Verification items for the finished model (mm, model axes). A direction names the side the tool comes from. Give positions to 0.01 mm unless a question says otherwise; leave off trailing zeros. Loops run counter-clockwise (first coordinate to the right, second up) from the corner with the lowest first, then second, coordinate; pieces in that order, holes last. Notation, with made-up numbers: M -39.5,-3 L 12.5,-3 A16 ccw 12.5,14 Z; hole C 11,21.5 d9. An arc over 180 degrees is marked long. Use CSV: the item, a comma, the result in double quotes.
from build123d import *

# Parameters (mm, degrees)
CROQUIS1_W              = 42
CROQUIS1_H              = 33.5
SALIENTE_EXTRUIR1_DEPTH = 5.5
SALIENTE_EXTRUIR2_DEPTH = 12
NERVIO4_REACH           = 72.794
CROQUIS4_WALL_W         = 160.558874412
CROQUIS4_WALL_H         = 8
CROQUIS5_R              = 4.5
CORTAR_EXTRUIR1_DEPTH   = 12
CROQUIS6_R              = 11.3
CORTAR_EXTRUIR2_DEPTH   = 9
CORTAR_EXTRUIR3_DEPTH   = 70.507193872
CHAFL_N1_SIZE           = 5


with BuildPart() as part:
    # Croquis1 → Saliente-Extruir1 (new, symmetric)
    with BuildSketch(Plane.XY):
        Rectangle(CROQUIS1_W, CROQUIS1_H)
        Polygon((21, -16.75), (-21, -16.75), (-45, -16.75), (-45, -33.25), (45, -33.25), (45, -16.75), align=None)
    extrude(amount=SALIENTE_EXTRUIR1_DEPTH, both=True)

    # Croquis2 → Saliente-Extruir2 (add)
    with BuildSketch(Plane.XY.offset(5.5)):
        Polygon((-21, -16.75), (-45, -16.75), (-45, -33.25), (45, -33.25), (45, -16.75), (21, -16.75), align=None)
    extrude(amount=SALIENTE_EXTRUIR2_DEPTH)

    # Croquis4 wall → Nervio4 (add, up to next)
    with BuildSketch(Plane(origin=(15, -10.75, 11.5), x_dir=(0, -0.707106781187, 0.707106781187), z_dir=(0, -0.707106781187, -0.707106781187)), mode=Mode.PRIVATE) as nervio4_sk1:
        Rectangle(CROQUIS4_WALL_W, CROQUIS4_WALL_H)
    nervio4_tool1 = extrude(nervio4_sk1.sketch, amount=NERVIO4_REACH, mode=Mode.PRIVATE) - part.part
    nervio4 = nervio4_tool1.solids().sort_by_distance((15, -10.75, 11.5))[0]
    add(nervio4)

    # Simetría1: Nervio4 across plane
    add(nervio4.mirror(Plane(origin=(0, 0, 0), x_dir=(0, 0, 1), z_dir=(1, 0, 0))))

    # Croquis5 → Cortar-Extruir1 (cut)
    with BuildSketch(Plane.XY.offset(5.5)):
        Circle(CROQUIS5_R)
    extrude(amount=-CORTAR_EXTRUIR1_DEPTH, mode=Mode.SUBTRACT)

    # Croquis6 → Cortar-Extruir2 (cut)
    with BuildSketch(Plane.XY.offset(5.5)):
        Circle(CROQUIS6_R)
    extrude(amount=-CORTAR_EXTRUIR2_DEPTH, mode=Mode.SUBTRACT)

    # Croquis7 → Cortar-Extruir3 (cut, through all)
    with BuildSketch(Plane.XZ.offset(33.25)):
        with BuildLine():
            Line((-38.5, 8.5), (-26.5, 8.5))
            ThreePointArc((-26.5, 8.5), (-24, 6), (-26.5, 3.5))
            Line((-26.5, 3.5), (-38.5, 3.5))
            ThreePointArc((-38.5, 3.5), (-41, 6), (-38.5, 8.5))
        make_face()
        with BuildLine():
            Line((38.5, 8.5), (26.5, 8.5))
            ThreePointArc((26.5, 8.5), (24, 6), (26.5, 3.5))
            Line((26.5, 3.5), (38.5, 3.5))
            ThreePointArc((38.5, 3.5), (41, 6), (38.5, 8.5))
        make_face()
    extrude(amount=-CORTAR_EXTRUIR3_DEPTH, mode=Mode.SUBTRACT)

    # Chaflán1
    chafl_n1_edges = [part.edges().sort_by_distance(p)[0] for p in [
        (-21, 16.75, 0),
        (21, 16.75, 0),
    ]]
    chamfer(chafl_n1_edges, length=CHAFL_N1_SIZE)


solid = part.part
(1) Section check C-C on z = 10.5. Record the cut outline in (x, y).
Calculated:
outline,"M -45,-33.25 L 45,-33.25 L 45,-16.75 L 19,-16.75 L 19,-9.75 L 11,-9.75 L 11,-16.75 L -11,-16.75 L -11,-9.75 L -19,-9.75 L -19,-16.75 L -45,-16.75 Z"
(2) Section check B-B on y = 0. Record the cut outline in (x, z).
Calculated:
outline,"M -21,-5.5 L -4.5,-5.5 L -4.5,-3.5 L -11.3,-3.5 L -11.3,5.5 L -21,5.5 Z; M 4.5,-5.5 L 21,-5.5 L 21,5.5 L 11.3,5.5 L 11.3,-3.5 L 4.5,-3.5 Z"
(3) Section check A-A on x = 33. Record the cut outline in (y, z), plus the area to 3 significant figures.
Calculated:
outline,"M -33.25,-5.5 L -16.75,-5.5 L -16.75,3.5 L -33.25,3.5 Z; M -33.25,8.5 L -16.75,8.5 L -16.75,17.5 L -33.25,17.5 Z"
area,"297 mm²"
(4) Mould release check, pull along Z, two halves, no side actions. Record for faces 5 (the flat face through (-1, -25, 17.5)), 6 (the flat face through (0, -16.75, 11)), 7 (the flat face through (32, -25, 3.5)), 8 (the cylindrical face through (41, -25, 6)): released by +Z, released by -Z, zero draft, split by the parting line, or undercut.
Calculated:
face 5,"released by +Z"
face 6,"zero draft"
face 7,"undercut"
face 8,"undercut"
(5) Section check D-D on y = -24. Record the cut outline in (x, z), plus the area to 3 significant figures.
Calculated:
outline,"M -45,-5.5 L 45,-5.5 L 45,17.5 L -45,17.5 Z; hole M -38.5,3.5 L -26.5,3.5 A2.5 ccw -26.5,8.5 L -38.5,8.5 A2.5 ccw Z; hole M 26.5,3.5 L 38.5,3.5 A2.5 ccw 38.5,8.5 L 26.5,8.5 A2.5 ccw Z"
area,"1,910 mm²"
(6) Scan lines: L1, parallel to Y at x = 0, z = 1.5; L2, parallel to X at y = -18, z = 6; L3, parallel to Y at x = 23, z = -2.5. Record each from-to range of solid material in increasing order. Write a range as from..to.
Calculated:
L1,"y = -33.25..-11.3, 11.3..16.75"
L2,"x = -45..-41, -24..24, 41..45"
L3,"y = -33.25..-16.75"
(7) Depth check by flat-ended pin: pin 1 Ø13 at (y, z) = (-9.5, 12.5) entering from +X; pin 2 Ø3.5 at (x, z) = (-5, 13) entering from +Y; pin 3 Ø2 at (y, z) = (-15.5, 10) entering from -X. Enter the tip coordinate at first touch or a pass-through.
Calculated:
pin 1,"stops at x = 19"
pin 2,"stops at y = -16.75"
pin 3,"stops at x = -19"
(8) Tool access check on faces 1 (the flat face through (-11, -13, 9)), 2 (the flat face through (-19, -13, 9)), 3 (the flat face through (21, -3, 0)), 4 (the flat face through (-33, -25, 8.5)). Record the directions out of +Z, -Z, +X, -X, +Y, -Y that give a thin tool (end or side, any length) a straight path to the whole face; none if there is none.
Calculated:
face 1,"+Z, +Y"
face 2,"+Z, -X, +Y"
face 3,"+Z, -Z, +X, +Y"
face 4,"+Y, -Y"
